from build123d import *

# Parameters (mm, degrees)
F0_W     = 76.2
F0_H     = 101.6
F1_DEPTH = 50.8
F3_R     = 3.175
F5_DEPTH = 6.35
F2_R     = 3.175
F6_DEPTH = 6.35
F4_R     = 5.715
F7_DEPTH = 6.35
F8_R     = 1.27


with BuildPart() as f1:
    # F0 (on Front) → F1 (new body)
    with BuildSketch(Plane.XZ):
        Rectangle(F0_W, F0_H)
    extrude(amount=F1_DEPTH)

    # F3 (on face) → F5 (join)
    with BuildSketch(Plane(origin=(-38.1, 0, 0), x_dir=(0, -1, 0), z_dir=(-1, 0, 0))):
        with Locations((25.4, -25.4)):
            Circle(F3_R)
    extrude(amount=F5_DEPTH)

    # F2 (on face) → F6 (join)
    with BuildSketch(Plane.YZ.offset(38.1)):
        with Locations((-25.4, -25.4)):
            Circle(F2_R)
    extrude(amount=F6_DEPTH)

    # F4 (on face) → F7 (join)
    with BuildSketch(Plane.XY.offset(50.8)):
        with Locations((0, -25.4)):
            Circle(F4_R)
    extrude(amount=F7_DEPTH)

    # F8
    f8_edges = [f1.edges().sort_by_distance(p)[0] for p in [
        (44.45, -28.575, -25.4),
        (-5.715, -25.4, 57.15),
        (-44.45, -22.225, -25.4),
    ]]
    fillet(f8_edges, radius=F8_R)


solid = f1.part
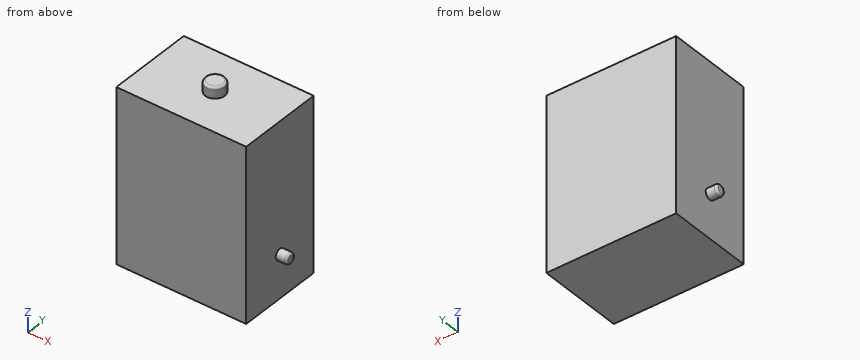
Geometry: final body of the model. Coordinates: model frame, mm. Coordinates: 2 decimals unless noted, no trailing zeros. Order: outer loops, then holes, each group sorted by start corner. A loop starts at its lowest first (then second) coordinate and runs counter-clockwise, first axis right, second up.
(1) Section query B-B (y = -25.4). Return the cut outline in (x, z) (3 decimals), plus the area to 3 significant figures.
(2) Material intervals for probe 1 along X at (y, z) = (-42.5, 0); probe 2 along Z at (x, y) = (26, -44), sorted ascending.
(3) Section query A-A (z = -25.4). Return the cut outline in (x, y) (3 decimals), plus the area to 3 significant figures.
(4) Section query C-C (x = 0). Return the cut outline in (y, z) (3 decimals).
(5) First-contact query: pin 1 (2 mm diameter, centred on y = -16.5, z = -1.5, fed in from -X); pin 2 (10 mm diameter, centred on y = -12.5, z = 29, fed in from +X); pin 3 (8 mm diameter, centred on x = 15.5, y = -31.5, fed in from +Z). Flat tips, straight axial feed; report the tip coordinate or a pass-through.
(6) Section query D-D (y = -44). Return the cut outline in (x, z), plus the area to 3 significant figures.
Solution:
1. outline: (-44.45, -27.305) arc R1.27 ccw to (-43.18, -28.575) - (-38.1, -28.575) - (-38.1, -50.8) - (38.1, -50.8) - (38.1, -28.575) - (43.18, -28.575) arc R1.27 ccw to (44.45, -27.305) - (44.45, -23.495) arc R1.27 ccw to (43.18, -22.225) - (38.1, -22.225) - (38.1, 50.8) - (5.715, 50.8) - (5.715, 55.88) arc R1.27 ccw to (4.445, 57.15) - (-4.445, 57.15) arc R1.27 ccw to (-5.715, 55.88) - (-5.715, 50.8) - (-38.1, 50.8) - (-38.1, -22.225) - (-43.18, -22.225) arc R1.27 ccw to (-44.45, -23.495) - close
1. area: 7,890 mm2
2. probe 1: x = -38.1 to 38.1
2. probe 2: z = -50.8 to 50.8
3. outline: (-44.45, -27.305) arc R1.27 ccw to (-43.18, -28.575) - (-38.1, -28.575) - (-38.1, -50.8) - (38.1, -50.8) - (38.1, -28.575) - (43.18, -28.575) arc R1.27 ccw to (44.45, -27.305) - (44.45, -23.495) arc R1.27 ccw to (43.18, -22.225) - (38.1, -22.225) - (38.1, 0) - (-38.1, 0) - (-38.1, -22.225) - (-43.18, -22.225) arc R1.27 ccw to (-44.45, -23.495) - close
3. area: 3,950 mm2
4. outline: (-50.8, -50.8) - (0, -50.8) - (0, 50.8) - (-19.685, 50.8) - (-19.685, 55.88) arc R1.27 ccw to (-20.955, 57.15) - (-29.845, 57.15) arc R1.27 ccw to (-31.115, 55.88) - (-31.115, 50.8) - (-50.8, 50.8) - close
5. pin 1: stops at x = -38.1
5. pin 2: stops at x = 38.1
5. pin 3: stops at z = 50.8
6. outline: (-38.1, -50.8) - (38.1, -50.8) - (38.1, 50.8) - (-38.1, 50.8) - close
6. area: 7,740 mm2
